```python
from build123d import *

# Parameters (mm, degrees)
BOSS_EXTRUDE1_DEPTH          = 2.5
TAP_DRILL_FOR_M12X1_5_TAP1_D = 12
HOLE1_D                      = 1.8
SKETCH7_R                    = 1.1
CUT_EXTRUDE1_DEPTH           = 33.805449556


with BuildPart() as part:
    # Sketch1 → Boss-Extrude1 (new, symmetric)
    with BuildSketch(Plane.XY):
        with BuildLine():
            Line((-31.542788725, 2.5), (-7.071067812, 2.5))
            ThreePointArc((-7.071067812, 2.5), (0.871651704, 7.449176015), (7.457211275, 0.8))
            Line((7.457211275, 0.8), (17.457211275, 0.8))
            Line((17.457211275, 0.8), (17.457211275, -0.8))
            Line((17.457211275, -0.8), (7.457211275, -0.8))
            ThreePointArc((7.457211275, -0.8), (0.871651704, -7.449176015), (-7.071067812, -2.5))
            Line((-7.071067812, -2.5), (-31.542788725, -2.5))
            Line((-31.542788725, -2.5), (-31.542788725, -0.8))
            Line((-31.542788725, -0.8), (-25.542788725, -0.8))
            Line((-25.542788725, -0.8), (-25.542788725, 0.8))
            Line((-25.542788725, 0.8), (-31.542788725, 0.8))
            Line((-31.542788725, 0.8), (-31.542788725, 2.5))
        make_face()
    extrude(amount=BOSS_EXTRUDE1_DEPTH, both=True)

    # Tap Drill for M12x1.5 Tap1 (through all)
    with Locations(Plane.XY.offset(2.5)):
        with Locations((0, 0)):
            Hole(TAP_DRILL_FOR_M12X1_5_TAP1_D / 2)

    # Hole1 (through all)
    with Locations(Plane(origin=(0, 2.5, 0), x_dir=(1, 0, 0), z_dir=(0, 1, 0))):
        with Locations((-28.542788725, 0)):
            Hole(HOLE1_D / 2)

    # Sketch7 → Cut-Extrude1 (cut, through all)
    with BuildSketch(Plane.XY.offset(-2.5)):
        with Locations((-8.25, 0)):
            Circle(SKETCH7_R)
        with Locations((-22.75, 0)):
            Circle(SKETCH7_R)
    extrude(amount=CUT_EXTRUDE1_DEPTH, mode=Mode.SUBTRACT)


solid = part.part
```
Could you check a few things on this model? Use its own coordinates, in mm. A direction names the side the tool comes from. Round coordinates to 2 decimals unless told otherwise and drop trailing zeros. Order: outer loops, then holes, each group sorted by start corner. A loop starts at its lowest first (then second) coordinate and runs counter-clockwise, first axis right, second up. Notation, with made-up numbers: (-28.75, -4) -> (23.25, -4) arc R16 ccw to (23.25, 25) -> close; hole circle Ø1 at (84.5, 6). An arc over 180 degrees is marked (long way). One line per question, with ' | ' between items.
Q1. Which directions (+Z, -Z, +X, -X, +Y, -Y) give clear straight access to the entire face, cutting with the end or side of a thin tool? Please do faces 1 (the face through (-28, 0.8, 1)), 2 (the face through (-19, -2.5, 0)), 3 (the face through (-19, 2.5, 0)), 4 (the face through (6, 0, 0)), 5 (the face through (13, -0.8, 0)).
Computed values:
face 1: +Z, -Z, -X | face 2: +Z, -Z, -X, -Y | face 3: +Z, -Z, -X, +Y | face 4: +Z, -Z | face 5: +Z, -Z, +X, -Y
Q2. If I drill on line 1 (Y direction, x = -22.75, z = 0.35); line 2 (X direction, y = -0.5, z = -1.75); line 3 (X direction, y = 1.75, z = 0.7), over which ranges is the centre line in solid material (lowest first)? Write a range as from..to.
Computed values:
line 1: -2.5..-1.1, 1.1..2.5 | line 2: -25.54..-23.73, -21.77..-9.23, -7.27..-5.98, 5.98..17.46 | line 3: -31.54..-29.11, -27.98..-5.74, 5.74..7.29
Q3. If we section it at D-D on z = -1.9: Write out the boundary of the cut face in (x, y), plus the area to 3 significant figures.
Computed values:
outline: (-31.54, -2.5) -> (-7.07, -2.5) arc R7.5 ccw to (7.46, -0.8) -> (17.46, -0.8) -> (17.46, 0.8) -> (7.46, 0.8) arc R7.5 ccw to (-7.07, 2.5) -> (-31.54, 2.5) -> (-31.54, 0.8) -> (-25.54, 0.8) -> (-25.54, -0.8) -> (-31.54, -0.8) -> close; hole circle Ø2.2 at (-22.75, 0); hole circle Ø2.2 at (-8.25, 0); hole circle Ø12 at (0, 0) | area: 183 mm²
Q4. If we section it at B-B on y = 0: Write out the boundary of the cut face in (x, z).
Computed values:
outline: (-25.54, -2.5) -> (-23.85, -2.5) -> (-23.85, 2.5) -> (-25.54, 2.5) -> close; (-21.65, -2.5) -> (-9.35, -2.5) -> (-9.35, 2.5) -> (-21.65, 2.5) -> close; (-7.15, -2.5) -> (-6, -2.5) -> (-6, 2.5) -> (-7.15, 2.5) -> close; (6, -2.5) -> (17.46, -2.5) -> (17.46, 2.5) -> (6, 2.5) -> close
Q5. I'm going to push flat-ended pins straight in: pin 1 (1.5 mm diameter, centred on x = -20.5, z = -1, fed in from +Y); pin 2 (2 mm diameter, centred on x = 4.5, z = 0, fed in from -Y); pin 3 (1.5 mm diameter, centred on x = 14, z = 0, fed in from -Y); pin 4 (1.4 mm diameter, centred on x = -28.54, z = 0, fed in from -Y). Where does each tip first touch, or does it pass through?
Computed values:
pin 1: y = 2.5 | pin 2: y = -6.63 | pin 3: y = -0.8 | pin 4: through
Q6. If we section it at A-A on z = 0: Write out the boundary of the cut face in (x, y), plus the area to 3 significant figures.
Computed values:
outline: (-31.54, -2.5) -> (-29.44, -2.5) -> (-29.44, -0.8) -> (-31.54, -0.8) -> close; (-31.54, 0.8) -> (-29.44, 0.8) -> (-29.44, 2.5) -> (-31.54, 2.5) -> close; (-27.64, -2.5) -> (-7.07, -2.5) arc R7.5 ccw to (7.46, -0.8) -> (17.46, -0.8) -> (17.46, 0.8) -> (7.46, 0.8) arc R7.5 ccw to (-7.07, 2.5) -> (-27.64, 2.5) -> (-27.64, 0.8) -> (-25.54, 0.8) -> (-25.54, -0.8) -> (-27.64, -0.8) -> close; hole circle Ø2.2 at (-22.75, 0); hole circle Ø2.2 at (-8.25, 0); hole circle Ø12 at (0, 0) | area: 177 mm²
Q7. If we section it at C-C on x = -8.25: Write out the boundary of the cut face in (y, z), plus the area to 3 significant figures.
Computed values:
outline: (-2.5, -2.5) -> (-1.1, -2.5) -> (-1.1, 2.5) -> (-2.5, 2.5) -> close; (1.1, -2.5) -> (2.5, -2.5) -> (2.5, 2.5) -> (1.1, 2.5) -> close | area: 14.0 mm²
Q8. We'd pull the mould along Y, two halves only. Please class faces 6 (the face through (12, 0.8, 0)), 7 (the face through (-29, -0.8, 1)), 8 (the face through (-11, 0, -2.5)): released by +Y, released by -Y, zero draft, split by the parting line, or undercut.
Computed values:
face 6: released by +Y | face 7: undercut | face 8: zero draft
